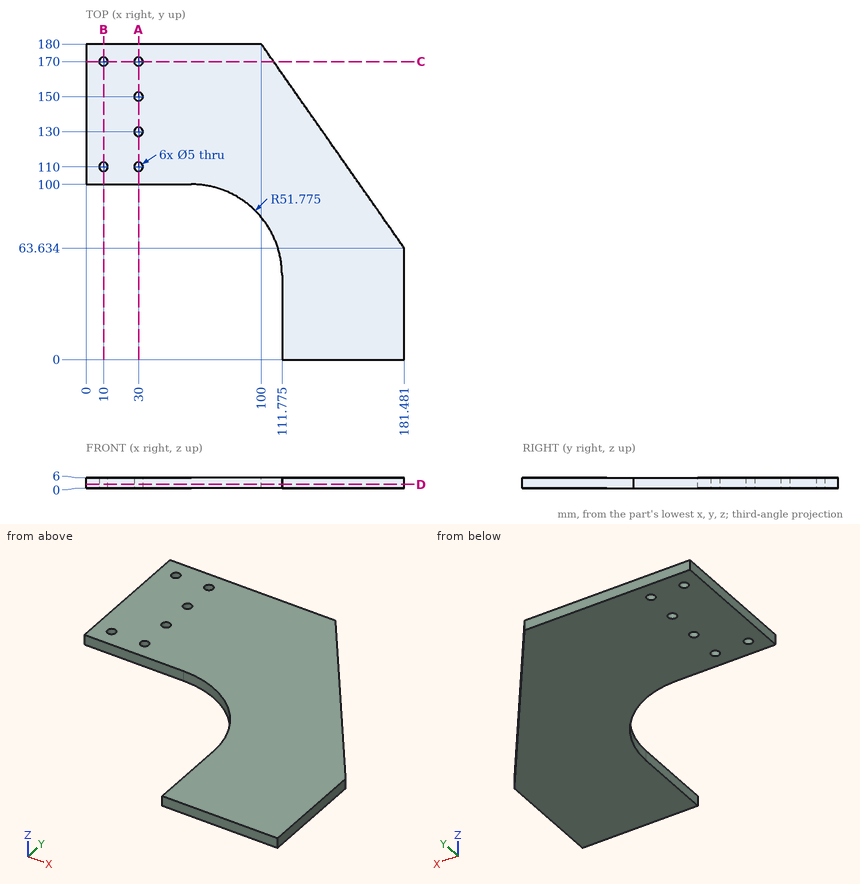
Geometry check sheet. Reference: drawing and pictorial views, mm from the part's lowest x, y, z. Coordinates: 2 decimals unless noted, no trailing zeros. Order: outer loops, then holes, each group sorted by start corner. A loop starts at its lowest first (then second) coordinate and runs counter-clockwise, first axis right, second up.
Item 1: Material ranges on L1, parallel to Y at x = 30, z = 4.4; L2, parallel to Y at x = 10, z = 4.75; L3, parallel to Y at x = 11.5, z = 2.95, recorded low to high.
Filled in:
L1: y = 100 to 107.5, 112.5 to 127.5, 132.5 to 147.5, 152.5 to 167.5, 172.5 to 180
L2: y = 100 to 107.5, 112.5 to 167.5, 172.5 to 180
L3: y = 100 to 108, 112 to 168, 172 to 180
Item 2: Depth check by flat-ended pin: pin 1 (2 mm diameter, centred on x = 23.5, z = 0.5, fed in from -Y); pin 2 (3 mm diameter, centred on y = 18.5, z = 2.5, fed in from -X) (1 decimal); pin 3 (3 mm diameter, centred on x = 119, y = 158, fed in from -Z). Enter the tip coordinate at first touch or a pass-through.
Filled in:
pin 1: stops at y = 100
pin 2: stops at x = 111.8
pin 3: passes through
Item 3: Section check A-A, the plane x = 30. Enter the section's corners in (y, z), then the cut area to 3 significant figures.
Filled in:
outline: (100, 0) - (107.5, 0) - (107.5, 6) - (100, 6) - close; (112.5, 0) - (127.5, 0) - (127.5, 6) - (112.5, 6) - close; (132.5, 0) - (147.5, 0) - (147.5, 6) - (132.5, 6) - close; (152.5, 0) - (167.5, 0) - (167.5, 6) - (152.5, 6) - close; (172.5, 0) - (180, 0) - (180, 6) - (172.5, 6) - close
area: 360 mm2
Item 4: Section check D-D, the plane z = 2.2. Give the number of separate pieces and of enclosed holes in the cut face, then the cut area to 3 significant figures.
Filled in:
separate pieces: 1
enclosed holes: 6
area: 17,200 mm2
Item 5: Section check C-C, the plane y = 170. Enter the section's corners in (x, z).
Filled in:
outline: (0, 0) - (7.5, 0) - (7.5, 6) - (0, 6) - close; (12.5, 0) - (27.5, 0) - (27.5, 6) - (12.5, 6) - close; (32.5, 0) - (107, 0) - (107, 6) - (32.5, 6) - close
Item 6: Section check B-B, the plane x = 10. Enter the section's corners in (y, z).
Filled in:
outline: (100, 0) - (107.5, 0) - (107.5, 6) - (100, 6) - close; (112.5, 0) - (167.5, 0) - (167.5, 6) - (112.5, 6) - close; (172.5, 0) - (180, 0) - (180, 6) - (172.5, 6) - close
